For this review, take the finished solid that the model builds, in its own axes (mm). Face numbers are marked on the shaded views. A direction names the side the tool comes from. Round coordinates to 2 decimals unless told otherwise and drop trailing zeros. Loops run counter-clockwise (first coordinate to the right, second up) from the corner with the lowest first, then second, coordinate; pieces in that order, holes last. Notation, with made-up numbers: M 32.5,35 L 42.5,35 A15 ccw 42.5,44 Z; hole C 30,-17 d3. An arc over 180 degrees is marked long. One line per question, with ' | ' between items. Start each with the question number.
1) We need section B-B (z = -13). State how many separate pieces and enclosed holes the cut face has, and give its area (3 significant figures).
2) For pin 1 Ø7.5 at (x, y) = (15, -7.24) entering from +Z; pin 2 Ø1.5 at (x, y) = (8.5, -13.5) entering from -Z; pin 3 Ø3.5 at (x, z) = (2, -10) entering from -Y, all flat-tipped, find the tip position at first contact; note any pin that passes through.
3) We need section D-D (x = 15). Give the boundary of the cut face in (y, z).
4) We need section A-A (y = 3.5). Give the boundary of the cut face in (x, z) (3 decimals).
5) For the marked faces 5, 6 and 7, list the 3-axis set-ups (+Z, -Z, +X, -X, +Y, -Y) from which the entire face can be reached by the end or side of a thin tool; tool diameter is ignored.
6) Mouldability with a two-part tool opening along X and no side actions: class the marked faces 1, 2, 3 and 4 as pulls with the +X half, pulls with the -X half, needs draft (parallel to the pull), parting line crosses it, or undercut.
7) For probe 1 along X at (y, z) = (-14.5, 7); probe 2 along Z at (x, y) = (22.5, -0.5); probe 3 along Z at (x, y) = (22.5, -8.25), list the stretches that pass through material, from the lowest coordinate up. Write a range as from..to.
```python
from build123d import *
from OCP.BRepFilletAPI import BRepFilletAPI_MakeChamfer

# Parameters (mm, degrees)
RESSALTO_EXTRUS_O1_DEPTH = 30
CORTE_EXTRUS_O1_REACH    = 49.448
ESBO_O2_R                = 2.375
ESBO_O2_R_2              = 3.25
ESBO_O2_3_R              = 4.75
ESBO_O2_3_R_2            = 2.375
CORTE_EXTRUS_O3_DEPTH    = 4
CORTE_EXTRUS_O2_REACH    = 54.89
ESBO_O3_R                = 2.375
ESBO_O3_3_R              = 2.375
CORTE_EXTRUS_O4_DEPTH    = 4
ESBO_O4_W                = 6
ESBO_O4_H                = 6
ESBO_O4_W_2              = 3
RESSALTO_EXTRUS_O2_DEPTH = 1
ESBO_O5_R                = 6.5
CORTE_EXTRUS_O5_DEPTH    = 42.848200707
CHANFRO1_SIZE            = 1
ESBO_O6_W                = 10
ESBO_O6_H                = 6
RESSALTO_EXTRUS_O3_DEPTH = 1
CHANFRO2_SIZE            = 0.5
CHANFRO2_SIZE_2          = 1


with BuildPart() as part:
    # Esboço1 → Ressalto-extrusão1 (new body)
    with BuildSketch(Plane(origin=(0, 0, 0), x_dir=(0, 0, -1), z_dir=(1, 0, 0))):
        Polygon((21.243161309, 12.755336939), (-18.756838691, 12.755336939), (-18.756838691, -9.981327227), (-11.493502857, -17.244663061), (1.243161309, -17.244663061), (1.243161309, 2.755336939), (21.243161309, 2.755336939), align=None)
    extrude(amount=RESSALTO_EXTRUS_O1_DEPTH)

    # Esboço2 → Corte-extrusão1 (cut, up to next)
    with BuildSketch(Plane(origin=(0, 12.755336939, 0), x_dir=(1, 0, 0), z_dir=(0, 1, 0)), mode=Mode.PRIVATE) as corte_extrus_o1_sk1:
        with Locations(Location((7.5, 11.243161309, 0), (0, 0, 270))):
            Circle(ESBO_O2_R)
    corte_extrus_o1_tool1 = extrude(corte_extrus_o1_sk1.sketch, amount=-CORTE_EXTRUS_O1_REACH, mode=Mode.PRIVATE) & part.part
    # Esboço2 → Corte-extrusão1 (cut, up to next)
    with BuildSketch(Plane(origin=(0, 12.755336939, 0), x_dir=(1, 0, 0), z_dir=(0, 1, 0)), mode=Mode.PRIVATE) as corte_extrus_o1_sk2:
        with Locations(Location((22.5, 11.243161309, 0), (0, 0, 270))):
            Circle(ESBO_O2_R)
    corte_extrus_o1_tool2 = extrude(corte_extrus_o1_sk2.sketch, amount=-CORTE_EXTRUS_O1_REACH, mode=Mode.PRIVATE) & part.part
    # Esboço2 → Corte-extrusão1 (cut, up to next)
    with BuildSketch(Plane(origin=(0, 12.755336939, 0), x_dir=(1, 0, 0), z_dir=(0, 1, 0)), mode=Mode.PRIVATE) as corte_extrus_o1_sk3:
        with Locations(Location((22.5, -7.256838691, 0), (0, 0, 270))):
            Circle(ESBO_O2_R_2)
    corte_extrus_o1_tool3 = extrude(corte_extrus_o1_sk3.sketch, amount=-CORTE_EXTRUS_O1_REACH, mode=Mode.PRIVATE) & part.part
    # Esboço2 → Corte-extrusão1 (cut, up to next)
    with BuildSketch(Plane(origin=(0, 12.755336939, 0), x_dir=(1, 0, 0), z_dir=(0, 1, 0)), mode=Mode.PRIVATE) as corte_extrus_o1_sk4:
        with Locations(Location((7.5, -7.256838691, 0), (0, 0, 270))):
            Circle(ESBO_O2_R_2)
    corte_extrus_o1_tool4 = extrude(corte_extrus_o1_sk4.sketch, amount=-CORTE_EXTRUS_O1_REACH, mode=Mode.PRIVATE) & part.part
    add(corte_extrus_o1_tool1.solids().sort_by_distance((7.5, 12.755337, -11.243161))[0], mode=Mode.SUBTRACT)
    add(corte_extrus_o1_tool2.solids().sort_by_distance((22.5, 12.755337, -11.243161))[0], mode=Mode.SUBTRACT)
    add(corte_extrus_o1_tool3.solids().sort_by_distance((22.5, 12.755337, 7.256839))[0], mode=Mode.SUBTRACT)
    add(corte_extrus_o1_tool4.solids().sort_by_distance((7.5, 12.755337, 7.256839))[0], mode=Mode.SUBTRACT)

    # Esboço2<3> → Corte-extrusão3 (cut)
    # profile 1 of 2: a face of its own
    with BuildSketch(Plane(origin=(0, 12.755336939, 0), x_dir=(1, 0, 0), z_dir=(0, 1, 0))):
        with Locations(Location((7.5, 11.243161309, 0), (0, 0, 270))):
            Circle(ESBO_O2_3_R)
        with Locations(Location((7.5, 11.243161309, 0), (0, 0, 270))):
            Circle(ESBO_O2_3_R_2, mode=Mode.SUBTRACT)
    # profile 2 of 2: a face of its own
    with BuildSketch(Plane(origin=(0, 12.755336939, 0), x_dir=(1, 0, 0), z_dir=(0, 1, 0))):
        with Locations(Location((22.5, 11.243161309, 0), (0, 0, 270))):
            Circle(ESBO_O2_3_R)
        with Locations(Location((22.5, 11.243161309, 0), (0, 0, 270))):
            Circle(ESBO_O2_3_R_2, mode=Mode.SUBTRACT)
    extrude(amount=-CORTE_EXTRUS_O3_DEPTH, mode=Mode.SUBTRACT)

    # Esboço3 → Corte-extrusão2 (cut, up to next)
    with BuildSketch(Plane.XY.offset(18.756838691), mode=Mode.PRIVATE) as corte_extrus_o2_sk1:
        with Locations((15, -7.244663061)):
            Circle(ESBO_O3_R)
    corte_extrus_o2_tool1 = extrude(corte_extrus_o2_sk1.sketch, amount=-CORTE_EXTRUS_O2_REACH, mode=Mode.PRIVATE) & part.part
    add(corte_extrus_o2_tool1.solids().sort_by_distance((15, -7.244663, 18.756839))[0], mode=Mode.SUBTRACT)

    # Esboço3<3> → Corte-extrusão4 (cut)
    # profile 1 of 2: a face of its own
    with BuildSketch(Plane.XY.offset(18.756838691)):
        with BuildLine():
            Line((18.882417963, -9.981327227), (11.117582037, -9.981327227))
            ThreePointArc((11.117582037, -9.981327227), (15, -11.994663061), (18.882417963, -9.981327227))
        make_face()
    # profile 2 of 2: a face of its own
    with BuildSketch(Plane.XY.offset(18.756838691)):
        with BuildLine():
            ThreePointArc((18.882417963, -9.981327227), (19.527912617, -8.680109799), (19.75, -7.244663061))
            ThreePointArc((19.75, -7.244663061), (13.564553262, -2.716750444), (11.117582037, -9.981327227))
            Line((11.117582037, -9.981327227), (18.882417963, -9.981327227))
        make_face()
        with Locations((15, -7.244663061)):
            Circle(ESBO_O3_3_R, mode=Mode.SUBTRACT)
    extrude(amount=-CORTE_EXTRUS_O4_DEPTH, mode=Mode.SUBTRACT)

    # Esboço4 → Ressalto-extrusão2 (add)
    with BuildSketch(Plane.XZ.offset(-2.755336939)):
        with Locations((15, -11.243161309)):
            Rectangle(ESBO_O4_W, ESBO_O4_H)
        with Locations((1.5, -11.243161309)):
            Rectangle(ESBO_O4_W_2, ESBO_O4_H)
        with Locations((28.5, -11.243161309)):
            Rectangle(ESBO_O4_W_2, ESBO_O4_H)
    extrude(amount=RESSALTO_EXTRUS_O2_DEPTH)

    # Esboço5 → Corte-extrusão5 (cut, through all)
    with BuildSketch(Plane.XZ.offset(-2.755336939)):
        with Locations(Location((7.5, 7.256838691, 0), (0, 0, 40.677035539))):
            Circle(ESBO_O5_R)
        with Locations(Location((22.5, 7.256838691, 0), (0, 0, 40.677035539))):
            Circle(ESBO_O5_R)
    extrude(amount=CORTE_EXTRUS_O5_DEPTH, mode=Mode.SUBTRACT)

    # Chanfro1
    chanfro1_edges = [part.edges().sort_by_distance(p)[0] for p in [
        (0, 12.755336939, -1.243161309),
        (30, 12.755336939, -1.243161309),
        (15, 12.755336939, 18.756838691),
        (15, 12.755336939, -21.243161309),
    ]]
    chamfer(chanfro1_edges, length=CHANFRO1_SIZE)

    # Esboço6 → Ressalto-extrusão3 (add)
    with BuildSketch(Plane(origin=(0, 0, -1.243161309), x_dir=(-1, 0, 0), z_dir=(0, 0, -1))):
        with Locations((-25, -7.244663061)):
            Rectangle(ESBO_O6_W, ESBO_O6_H)
        with Locations((-5, -7.244663061)):
            Rectangle(ESBO_O6_W, ESBO_O6_H)
    extrude(amount=RESSALTO_EXTRUS_O3_DEPTH)

    # Chanfro2
    chanfro2_edges_1 = [part.edges().sort_by_distance(p)[0] for p in [
        (25, -4.244663061, -1.243161309),
    ]]
    chanfro2_side_1 = [part.faces().sort_by_distance(p)[0] for p in [
        (25, -4.234663061, -1.243161309),
    ]]
    chanfro2_edges_2 = [part.edges().sort_by_distance(p)[0] for p in [
        (5, -4.244663061, -1.243161309),
    ]]
    chanfro2_side_2 = [part.faces().sort_by_distance(p)[0] for p in [
        (5, -4.234663061, -1.243161309),
    ]]
    chanfro2 = BRepFilletAPI_MakeChamfer(part.part.solid().wrapped)
    for e in chanfro2_edges_1:
        chanfro2.Add(CHANFRO2_SIZE - 0.0001, CHANFRO2_SIZE_2 - 0.0001, e.wrapped, chanfro2_side_1[0].wrapped)
    for e in chanfro2_edges_2:
        chanfro2.Add(CHANFRO2_SIZE - 0.0001, CHANFRO2_SIZE_2 - 0.0001, e.wrapped, chanfro2_side_2[0].wrapped)
    add(Compound.cast(chanfro2.Shape()), mode=Mode.REPLACE)  # a hair under: the kernel refuses the full size


solid = part.part
```
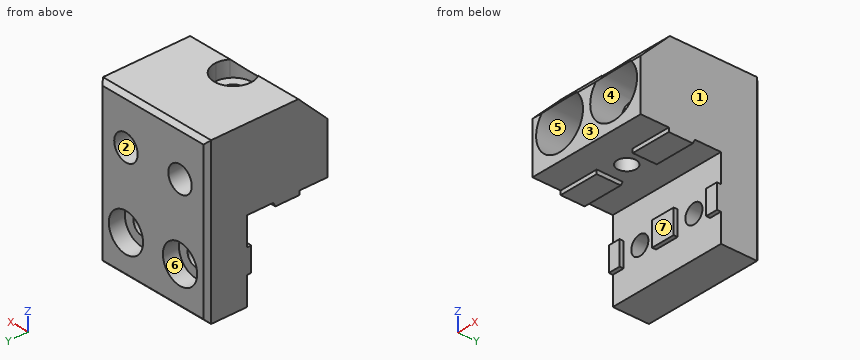
Answers below:
1) separate pieces: 3 | enclosed holes: 0 | area: 202 mm^2
2) pin 1: z = 14.76 | pin 2: z = -1.24 | pin 3: y = 1.76
3) outline: M -17.24,-1.24 L -9.62,-1.24 L -9.62,14.76 L -11.99,14.76 L -11.99,16.74 L -17.24,11.49 Z; M -4.87,-1.24 L 2.76,-1.24 L 2.76,-8.24 L 1.76,-8.24 L 1.76,-14.24 L 2.76,-14.24 L 2.76,-21.24 L 11.76,-21.24 L 12.76,-20.24 L 12.76,17.76 L 11.76,18.76 L -2.49,18.76 L -2.49,14.76 L -4.87,14.76 Z
4) outline: M 0,-21.243 L 30,-21.243 L 30,18.757 L 0,18.757 Z; hole C 7.5,7.257 d6.5; hole C 7.5,-11.243 d4.75; hole C 22.5,7.257 d6.5; hole C 22.5,-11.243 d4.75
5) face 5: -Y | face 6: +Y | face 7: -Z, +X, -X, -Y
6) face 1: pulls with the +X half | face 2: undercut | face 3: needs draft | face 4: undercut
7) probe 1: 0..1.01, 13.99..16.01, 28.99..30 | probe 2: -1.24..0.76, 13.76..18.76 | probe 3: -2.24..0.76, 13.76..18.76
